Geometry check sheet. Reference: the model listing, model coordinates, mm. A direction names the side the tool comes from. Coordinates: 2 decimals unless noted, no trailing zeros. Loops run counter-clockwise (first coordinate to the right, second up) from the corner with the lowest first, then second, coordinate; pieces in that order, holes last. Notation, with made-up numbers: (70.25, -3.75) - (110.25, -3.75) arc R19 ccw to (110.25, 22.25) - close; hole circle Ø11 at (-22.5, 7). An arc over 180 degrees is marked (long way). One line per item, written item: value.
from build123d import *

# Parameters (mm, degrees)
F0_R     = 3
F1_DEPTH = 10
F2_R     = 3
F3_DEPTH = 5
F5_DEPTH = 24.001


with BuildPart() as f1:
    # F0 (on Top) → F1 (new body)
    with BuildSketch(Plane.XY):
        with BuildLine():
            Line((0, 24), (0, 0))
            Line((0, 0), (40, 0))
            Line((40, 0), (40, 8))
            Line((40, 8), (23, 8))
            ThreePointArc((23, 8), (19, 12), (23, 16))
            Line((23, 16), (40, 16))
            Line((40, 16), (40, 24))
            Line((40, 24), (0, 24))
        make_face()
        with Locations((9.5, 12)):
            Circle(F0_R, mode=Mode.SUBTRACT)
    extrude(amount=F1_DEPTH)

    # F2 (on face) → F3 (cut)
    with BuildSketch(Plane(origin=(0, 0, 0), x_dir=(1, 0, 0), z_dir=(0, 0, -1))):
        Polygon((9.5, -16.618802), (13.5, -14.309401), (13.5, -9.690599), (9.5, -7.381198), (5.5, -9.690599), (5.5, -14.309401), align=None)
        with Locations((9.5, -12)):
            Circle(F2_R, mode=Mode.SUBTRACT)
    extrude(amount=-F3_DEPTH, mode=Mode.SUBTRACT)

    # F4 (on face) → F5 (cut, through all)
    with BuildSketch(Plane.XZ):
        with BuildLine():
            Line((0, 10), (0, 0))
            ThreePointArc((0, 0), (2.928932, 7.071068), (10, 10))
            Line((10, 10), (0, 10))
        make_face()
        with BuildLine():
            Line((35.5, 6), (40, 1.5))
            Line((40, 1.5), (40, 10))
            Line((40, 10), (10, 10))
            ThreePointArc((10, 10), (14.472136, 8.944272), (18, 6))
            Line((18, 6), (35.5, 6))
        make_face()
    extrude(amount=-F5_DEPTH, mode=Mode.SUBTRACT)


solid = f1.part
(1) Go/stop test with flat-tipped pins: pin 1 Ø2.5 at (x, y) = (8, 12.5) entering from -Z; pin 2 Ø5 at (y, z) = (11.5, 3.5) entering from +X. Record where each tip stops, or that it passes through.
Reply:
pin 1: through
pin 2: x = 20.35
(2) Material ranges on probe 1 along Y at (x, z) = (27.5, 2.75); probe 2 along Y at (x, z) = (9.5, 8.5); probe 3 along X at (y, z) = (12, 6.7), recorded low to high. Write a range as from..to.
Reply:
probe 1: 0..8, 16..24
probe 2: 0..9, 15..24
probe 3: 2.58..6.5, 12.5..17.42
(3) Access from +Z, -Z, +X, -X, +Y, -Y to the whole of each face (thin tool, end or side, straight path). Record for faces 1 (the face through (20, 15, 0)), 2 (the face through (12.27, 10.85, 7.47)), 3 (the face through (13.5, 12, 2)), 4 (the face through (32, 8, 3)), 5 (the face through (27, 6, 6)).
Reply:
face 1: -Z, +X, -X, +Y, -Y
face 2: +Z, -Z
face 3: -Z
face 4: +Z, -Z, +X
face 5: +Z, +X, +Y, -Y
(4) Cross-section at B-B on x = 7.5. Record the cut outline in (y, z), and give its area (3 significant figures).
Reply:
outline: (0, 0) - (8.54, 0) - (8.54, 5) - (9.76, 5) - (9.76, 9.68) - (0, 9.68) - close; (14.24, 5) - (15.46, 5) - (15.46, 0) - (24, 0) - (24, 9.68) - (14.24, 9.68) - close
area: 177 mm2
(5) Cross-section at C-C on y = 13. Record the cut outline in (x, z), and give its area (3 significant figures).
Reply:
outline: (0, 0) - (5.5, 0) - (5.5, 5) - (6.67, 5) - (6.67, 9.43) arc R10 ccw to start; (12.33, 5) - (13.5, 5) - (13.5, 0) - (19.13, 0) - (19.13, 6) - (18, 6) arc R10 ccw to (12.33, 9.73) - close
area: 88.2 mm2
(6) Cross-section at D-D on y = 3. Record the cut outline in (x, z).
Reply:
outline: (0, 0) - (40, 0) - (40, 1.5) - (35.5, 6) - (18, 6) arc R10 ccw to (10, 10) arc R10 ccw to start
(7) Cross-section at A-A on z = 8. Record the cut outline in (x, y), and give its area (3 significant figures).
Reply:
outline: (4, 0) - (16, 0) - (16, 24) - (4, 24) - close; hole circle Ø6 at (9.5, 12)
area: 260 mm2
(8) Release check for a two-part mould opening along X. For faces 6 (the face through (37.7, 19.9, 3.8)), 7 (the face through (16, 24, 4)), 8 (the face through (11.47, 15.48, 2.46)) record: pulls with the +X half, pulls with the -X half, needs draft (parallel to the pull), parting line crosses it, or undercut.
Reply:
face 6: pulls with the +X half
face 7: needs draft
face 8: undercut
